Autodesk Inventor part; units mm, degrees
ref_plane "Work Plane1" through (0, 18, 0) normal (0, 1, 0) x (1, 0, 0)
ref_plane "YZ Plane" through (0, 0, 0) normal (1, 0, 0) x (0, 1, 0)
ref_plane "XZ Plane" through (0, 0, 0) normal (0, 1, 0) x (-1, 0, 0)
sketch "Sketch1" plane through (0, 0, 0) normal (0, 1, 0) x (-1, 0, 0)
  circle A0 centre (0, 0) radius 30
  dimension "d0" = 60
extrude "Extrusion1" add sketch "Sketch1" along normal blind 3
ref_plane "Work Plane1" through (0, 18, 0) normal (0, 1, 0) x (1, 0, 0)
sketch "Sketch2" plane through (0, 18, 0) normal (0, 1, 0) x (1, 0, 0)
  circle A0 centre (0, 0) radius 5
  dimension "d5" = 10
loft "Loft1" add profiles "Sketch2" section 1 edges at (30, 3, 0)
sketch "Sketch3" plane through (0, 0, 0) normal (0, -1, 0) x (1, 0, 0)
  circle A0 centre (0, 0) radius 5
  dimension "d10" = 10
extrude "Extrusion2" cut sketch "Sketch3" against normal blind 8
sketch "Sketch5" plane through (0, 18, 0) normal (0, 1, 0) x (1, 0, 0)
  circle A0 centre (0, 0) radius 2.75
  dimension "d16" = 5.5
extrude "Extrusion4" cut sketch "Sketch5" against normal through all
sketch "Sketch6" plane through (0, 18, 0) normal (0, 1, 0) x (1, 0, 0)
  line L0 (0, 4.6188) -> (4, 2.3094)
  line L1 (4, 2.3094) -> (4, -2.3094)
  line L2 (4, -2.3094) -> (0, -4.6188)
  line L3 (0, -4.6188) -> (-4, -2.3094)
  line L4 (-4, -2.3094) -> (-4, 2.3094)
  line L5 (-4, 2.3094) -> (0, 4.6188)
  point P0 (0, 0)
  point P1 (0, 0)
  dimension "d19" = 8
extrude "Extrusion5" cut sketch "Sketch6" against normal blind 4
properties part number "Bottom_Foot"
Check sheet for the modelled part. Datum: model origin and axes. Units: mm. A direction names the side the tool comes from. Coordinates: 2 decimals unless noted, no trailing zeros. Loops run counter-clockwise (first coordinate to the right, second up) from the corner with the lowest first, then second, coordinate; pieces in that order, holes last.
1) Access from +Z, -Z, +X, -X, +Y, -Y to the whole of each face (thin tool, end or side, straight path). Record for faces 1 (the face through (-2.028, 16.028, -3.448)), 2 (the face through (-0.596, 11.042, 2.685)), 3 (the face through (-1.08, 3.94, -4.88)).
2) Material ranges on probe 1 along X at (y, z) = (10.8, 0); probe 2 along X at (y, z) = (9.6, 0); probe 3 along Z at (x, y) = (2, 6.5), recorded low to high.
3) Sectioned sample at B-B (y = 5.25). Record the boundary of the cut face in (x, z).
4) Sectioned sample at C-C (y = 10.75). Record the boundary of the cut face in (x, z).
5) Sectioned sample at A-A (y = 16.5). Record the boundary of the cut face in (x, z), and give its area (3 significant figures).
6) Gauge pin test, flat ends, axial feed: pin 1 (9 mm diameter, centred on x = 0, z = 0, fed in from +Y); pin 2 (12 mm diameter, centred on x = -14, z = -2.5, fed in from +Y); pin 3 (6.5 mm diameter, centred on x = 0, z = 0.5, fed in from +Y); pin 4 (2 mm diameter, centred on x = 13.5, z = 19, fed in from +Y). Record the tip position at first contact, or that the pin passes through.
7) Release check for a two-part mould opening along X. For faces 4 (the face through (0, 0, -6)), 5 (the face through (-1.97, 16.03, 3.48)), 6 (the face through (29.97, 1.48, -1.32)) record: released by +X, released by -X, zero draft, split by the parting line, or undercut.
Check sheet entries:
1. face 1: +Y
1. face 2: +Y, -Y
1. face 3: -Y
2. probe 1: x = -17 to -2.75, 2.75 to 17
2. probe 2: x = -19 to -2.75, 2.75 to 19
2. probe 3: z = -24.08 to -4.58, 4.58 to 24.08
3. outline: circle Ø52.5 at (0, 0); hole circle Ø10 at (0, 0)
4. outline: circle Ø34.17 at (0, 0); hole circle Ø5.5 at (0, 0)
5. outline: circle Ø15 at (0, 0); hole (-4, -2.31) - (0, -4.62) - (4, -2.31) - (4, 2.31) - (0, 4.62) - (-4, 2.31) - close
5. area: 121 mm2
6. pin 1: stops at y = 18
6. pin 2: stops at y = 16.07
6. pin 3: stops at y = 14
6. pin 4: stops at y = 7.62
7. face 4: zero draft
7. face 5: undercut
7. face 6: split by the parting line
